Can you work these out from the model? Positions are in its coordinate system, mm. A direction names the side the tool comes from. Coordinates: 2 decimals unless noted, no trailing zeros. Loops run counter-clockwise (first coordinate to the right, second up) from the corner with the lowest first, then second, coordinate; pieces in that order, holes last. Notation, with made-up numbers: (64, 41.25) -> (109, 41.25) arc R22 cw to (109, 63.25) -> close; hole circle Ø2 at (5, -26). An arc over 180 degrees is marked (long way). Use one line per item in the form item = value. Start each with the question number.
(1) Imagine slicing it at D-D (x = -7.5). List the corners of the cut face in (y, z) for me.
(2) On a 3-axis mill with a long thin cutter (end or side, diameter ignored), from which of +Z, -Z, +X, -X, +Y, -Y can I reach the whole of each face in a straight line? I mean faces 1 (the flat face through (16, -5, 4)), 2 (the flat face through (-19, -15, 4)), 3 (the flat face through (-1.45, 5, 4)). Say none if no direction works.
(3) I'm going to push a flat-ended pin straight in: pin 1 (1 mm diameter, centred on x = -16, z = 3, fed in from -Y). Where does the tip first touch, or does it pass through?
(4) I need wall thicknesses on line 1 (X direction, y = -13, z = 1.75); line 2 (X direction, y = -12, z = 1); line 3 (X direction, y = 7.5, z = 4.75). Which ranges of each line are inside material? Lowest first, please. Write a range as [from, to].
(5) Imagine slicing it at C-C (y = 4.75). List the corners of the cut face in (x, z) for me, plus the area to 3 significant figures.
(6) Imagine slicing it at B-B (z = 2.75). List the corners of the cut face in (x, y) for me.
(7) Imagine slicing it at A-A (y = -6.25). List the corners of the cut face in (x, z) for me.
(8) Thinking about a two-plate mould opening in X: for faces 4 (the flat face through (-17.15, -10, 4)), 5 (the flat face through (10, -15, 4)), 6 (the flat face through (4, -5, 4)), 7 (the flat face through (-20.15, -1, 4)), which applies, released by +X, released by -X, zero draft, split by the parting line, or undercut?
```python
from build123d import *

# Parameters (mm, degrees)
BOSS_EXTRUDE1_DEPTH = 8
FILLET6_R           = 2
FILLET7_R           = 2
FILLET8_R           = 2


with BuildPart() as part:
    # Sketch1 → Boss-Extrude1 (new body)
    with BuildSketch(Plane.XY):
        Polygon((-17.15, -15), (-17.15, -5), (-15.05, -5), (-15.05, -15), (2.95, -15), (2.95, -5), (5.05, -5), (5.05, -15), (15.05, -15), (15.05, -5), (17.15, -5), (17.15, -15), (20.15, -15), (20.15, 15), (-20.15, 15), (-20.15, -15), align=None)
        Polygon((-1.4497978, 7.740960344), (-6.4897978, 10.650805701), (-11.5297978, 7.740960344), (-11.5297978, 1.921269631), (-6.4897978, -0.988575726), (-1.4497978, 1.921269631), align=None, mode=Mode.SUBTRACT)
    extrude(amount=BOSS_EXTRUDE1_DEPTH)

    # Fillet6
    fillet6_edges = [part.edges().sort_by_distance(p)[0] for p in [
        (-20.15, 15, 4),
    ]]
    fillet(fillet6_edges, radius=FILLET6_R)

    # Fillet7
    fillet7_edges = [part.edges().sort_by_distance(p)[0] for p in [
        (20.15, 0, 0),
        (20.15, 15, 4),
        (20.15, 0, 8),
    ]]
    fillet(fillet7_edges, radius=FILLET7_R)

    # Fillet8
    # the kernel refuses this fillet: 2 mm, written as the material it takes off along each edge
    with BuildSketch(Plane(origin=(18.15, 13, 2), x_dir=(0, 0, -1), z_dir=(0, 1, 0))) as fillet8_piece_1_section:
        Polygon((0, 0), (FILLET8_R, 0), (FILLET8_R, -FILLET8_R), (0, -FILLET8_R), align=None)
    fillet8_piece_1 = extrude(amount=FILLET8_R, mode=Mode.PRIVATE)
    fillet8_piece_1 = fillet8_piece_1 - Plane(origin=(18.15, 13, 2), x_dir=(-0.7071067811865475, 0, 0.7071067811865475), z_dir=(0, 1, 0)) * Sphere(FILLET8_R, mode=Mode.PRIVATE)
    add(fillet8_piece_1, mode=Mode.SUBTRACT)
    with BuildSketch(Plane(origin=(18.15, 13, 6), x_dir=(0, 0, 1), z_dir=(0, 1, 0))) as fillet8_piece_2_section:
        Polygon((0, 0), (FILLET8_R, 0), (FILLET8_R, FILLET8_R), (0, FILLET8_R), align=None)
    fillet8_piece_2 = extrude(amount=FILLET8_R, mode=Mode.PRIVATE)
    fillet8_piece_2 = fillet8_piece_2 - Plane(origin=(18.15, 13, 6), x_dir=(-0.7071067811865475, 0, -0.7071067811865475), z_dir=(0, 1, 0)) * Sphere(FILLET8_R, mode=Mode.PRIVATE)
    add(fillet8_piece_2, mode=Mode.SUBTRACT)
    with BuildSketch(Plane(origin=(-20.15, 13, 0), x_dir=(1, 0, 0), z_dir=(0, -1, 0))) as fillet8_piece_3:
        with BuildLine():
            CenterArc((FILLET8_R, FILLET8_R), FILLET8_R, 180, 90)
            Line((0, FILLET8_R), (0, 0))
            Line((0, 0), (FILLET8_R, 0))
        make_face()
    extrude(amount=33, mode=Mode.SUBTRACT)
    with BuildSketch(Plane(origin=(-20.15, 13, 8), x_dir=(1, 0, 0), z_dir=(0, -1, 0))) as fillet8_piece_4:
        with BuildLine():
            CenterArc((FILLET8_R, -FILLET8_R), FILLET8_R, 90, 90)
            Line((0, -FILLET8_R), (0, 0))
            Line((0, 0), (FILLET8_R, 0))
        make_face()
    extrude(amount=33, mode=Mode.SUBTRACT)
    with BuildSketch(Plane(origin=(-18.15, 13, 0), x_dir=(0, 1, 0), z_dir=(1, 0, 0))) as fillet8_piece_5:
        with BuildLine():
            CenterArc((2 - FILLET8_R, FILLET8_R), FILLET8_R, 270, 90)
            Line((2, FILLET8_R), (2, 0))
            Line((2, 0), (2 - FILLET8_R, 0))
        make_face()
    revolve(axis=Axis((-18.15, 13, 0), (0, 0, 1)), revolution_arc=90, mode=Mode.SUBTRACT)
    with BuildSketch(Plane(origin=(-18.15, 13, 8), x_dir=(0, 1, 0), z_dir=(1, 0, 0))) as fillet8_piece_6:
        with BuildLine():
            CenterArc((2 - FILLET8_R, -FILLET8_R), FILLET8_R, 0, 90)
            Line((2 - FILLET8_R, 0), (2, 0))
            Line((2, 0), (2, -FILLET8_R))
        make_face()
    revolve(axis=Axis((-18.15, 13, 8), (0, 0, 1)), revolution_arc=90, mode=Mode.SUBTRACT)
    with BuildSketch(Plane(origin=(18.15, 15, 8), x_dir=(0, 0, -1), z_dir=(-1, 0, 0))) as fillet8_piece_7:
        with BuildLine():
            CenterArc((FILLET8_R, FILLET8_R), FILLET8_R, 180, 90)
            Line((0, FILLET8_R), (0, 0))
            Line((0, 0), (FILLET8_R, 0))
        make_face()
    extrude(amount=36.3, mode=Mode.SUBTRACT)
    with BuildSketch(Plane(origin=(18.15, 15, 0), x_dir=(0, 0, 1), z_dir=(-1, 0, 0))) as fillet8_piece_8:
        with BuildLine():
            CenterArc((FILLET8_R, -FILLET8_R), FILLET8_R, 90, 90)
            Line((0, -FILLET8_R), (0, 0))
            Line((0, 0), (FILLET8_R, 0))
        make_face()
    extrude(amount=36.3, mode=Mode.SUBTRACT)


solid = part.part
```
Worked out:
q1.outline = (-15, 0) -> (-0.41, 0) -> (-0.41, 8) -> (-15, 8) -> close; (10.07, 0) -> (13, 0) arc R2 ccw to (15, 2) -> (15, 6) arc R2 ccw to (13, 8) -> (10.07, 8) -> close
q2.face_1 = +Z, -Z, -Y
q2.face_2 = +Z, -Z, +X, -X, -Y
q2.face_3 = +Z, -Z
q3.pin_1 = -5
q4.line_1 = [-20.13, -17.15], [-15.05, 2.95], [5.05, 15.05], [17.15, 20.13]
q4.line_2 = [-19.88, -17.15], [-15.05, 2.95], [5.05, 15.05], [17.15, 19.88]
q4.line_3 = [-20.15, -11.53], [-1.45, 20.15]
q5.outline = (-20.15, 2) arc R2 ccw to (-18.15, 0) -> (-11.53, 0) -> (-11.53, 8) -> (-18.15, 8) arc R2 ccw to (-20.15, 6) -> close; (-1.45, 0) -> (18.15, 0) arc R2 ccw to (20.15, 2) -> (20.15, 6) arc R2 ccw to (18.15, 8) -> (-1.45, 8) -> close
q5.area = 238 mm2
q6.outline = (-20.15, -15) -> (-17.15, -15) -> (-17.15, -5) -> (-15.05, -5) -> (-15.05, -15) -> (2.95, -15) -> (2.95, -5) -> (5.05, -5) -> (5.05, -15) -> (15.05, -15) -> (15.05, -5) -> (17.15, -5) -> (17.15, -15) -> (20.15, -15) -> (20.15, 13) arc R2 ccw to (18.15, 15) -> (-18.15, 15) arc R2 ccw to (-20.15, 13) -> close; hole (-11.53, 1.92) -> (-6.49, -0.99) -> (-1.45, 1.92) -> (-1.45, 7.74) -> (-6.49, 10.65) -> (-11.53, 7.74) -> close
q7.outline = (-20.15, 2) arc R2 ccw to (-18.15, 0) -> (-17.15, 0) -> (-17.15, 8) -> (-18.15, 8) arc R2 ccw to (-20.15, 6) -> close; (-15.05, 0) -> (2.95, 0) -> (2.95, 8) -> (-15.05, 8) -> close; (5.05, 0) -> (15.05, 0) -> (15.05, 8) -> (5.05, 8) -> close; (17.15, 0) -> (18.15, 0) arc R2 ccw to (20.15, 2) -> (20.15, 6) arc R2 ccw to (18.15, 8) -> (17.15, 8) -> close
q8.face_4 = undercut
q8.face_5 = zero draft
q8.face_6 = undercut
q8.face_7 = released by -X
